Could you check a few things on this drawing? It's one solid part, dimensions in mm from its lowest x, y, z. Coordinates: 2 decimals unless noted, no trailing zeros. Write each loop counter-clockwise with the first axis right and the second up, starting at its lowest first coordinate (ties: lowest second). Pieces come first, ordered by that corner, then holes.
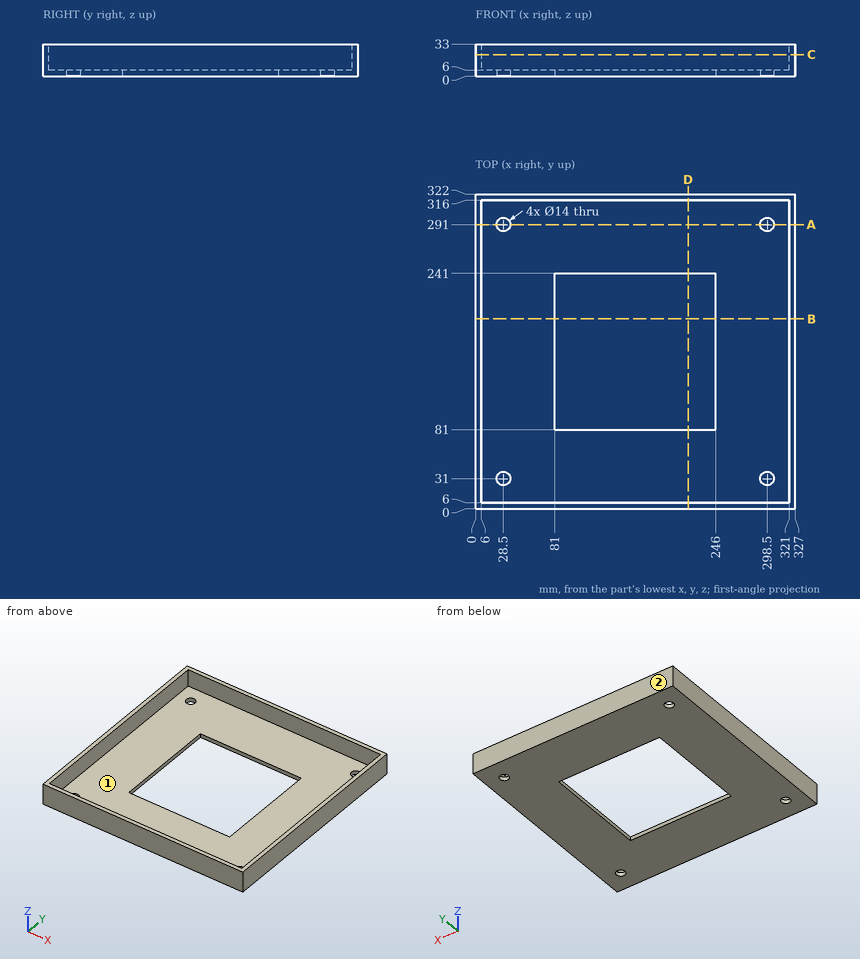
1) Imagine slicing it at C-C on z = 22. Please give me the cut outline in (x, y), then the cut area to 3 significant figures.
Values follow:
outline: (0, 0) - (327, 0) - (327, 322) - (0, 322) - close; hole (6, 6) - (321, 6) - (321, 316) - (6, 316) - close
area: 7,640 mm2
2) Imagine slicing it at B-B on y = 194.5. Please give me the cut outline in (x, z).
Values follow:
outline: (0, 0) - (81, 0) - (81, 6) - (6, 6) - (6, 33) - (0, 33) - close; (246, 0) - (327, 0) - (327, 33) - (321, 33) - (321, 6) - (246, 6) - close
3) Imagine slicing it at A-A on y = 291. Please give me the cut outline in (x, z), then the cut area to 3 significant figures.
Values follow:
outline: (0, 0) - (21.5, 0) - (21.5, 6) - (6, 6) - (6, 33) - (0, 33) - close; (35.5, 0) - (291.5, 0) - (291.5, 6) - (35.5, 6) - close; (305.5, 0) - (327, 0) - (327, 33) - (321, 33) - (321, 6) - (305.5, 6) - close
area: 2,120 mm2
4) We'd pull the mould along X, two halves only. Please class the marked faces 1 and 2: pulls with the +X half, pulls with the -X half, needs draft (parallel to the pull), parting line crosses it, or undercut.
Values follow:
face 1: undercut
face 2: needs draft
5) I need wall thicknesses on probe 1 along Y at (x, z) = (298, 1); probe 2 along X at (y, z) = (291, 1); probe 3 along X at (y, z) = (306, 21). Which ranges of each line are inside material? Lowest first, please.
Values follow:
probe 1: y = 0 to 24.02, 37.98 to 284.02, 297.98 to 322
probe 2: x = 0 to 21.5, 35.5 to 291.5, 305.5 to 327
probe 3: x = 0 to 6, 321 to 327
6) Will this pin go through, and if not, where does the flat tip stop? pin 1 (16 mm diameter, centred on x = 298.5, y = 291, fed in from +Z).
Values follow:
pin 1: stops at z = 6
7) Imagine slicing it at D-D on x = 217.5. Please give me the cut outline in (y, z).
Values follow:
outline: (0, 0) - (81, 0) - (81, 6) - (6, 6) - (6, 33) - (0, 33) - close; (241, 0) - (322, 0) - (322, 33) - (316, 33) - (316, 6) - (241, 6) - close
